```python
from build123d import *

# Parameters (mm, degrees)
SKETCH1_W                                    = 225
SKETCH1_H                                    = 47
SKETCH1_H_2                                  = 7
BOSS_EXTRUDE1_DEPTH                          = 3
SKETCH3_R                                    = 1.767766953
CUT_EXTRUDE1_DEPTH                           = 117.59974271
CHAMFER2_SIZE                                = 2
SKETCH2_W                                    = 225
SKETCH2_H                                    = 33
SKETCH2_R                                    = 15
CUT_EXTRUDE2_DEPTH                           = 0.2
FILLET1_R                                    = 3.5
CSK_FOR_M3_COUNTERSUNK_FLAT_HEAD_SCR_2_COUNT = 2
CSK_FOR_M3_COUNTERSUNK_FLAT_HEAD_SCR_2_PITCH = 47
CSK_FOR_M3_COUNTERSUNK_FLAT_HEAD_SCR_3_COUNT = 2
CSK_FOR_M3_COUNTERSUNK_FLAT_HEAD_SCR_3_PITCH = 223.00896843
CSK_FOR_M3_COUNTERSUNK_FLAT_HEAD_SCR_4_COUNT = 2
CSK_FOR_M3_COUNTERSUNK_FLAT_HEAD_SCR_4_PITCH = 218


with BuildPart() as part:
    # Sketch1 → Boss-Extrude1 (new body)
    with BuildSketch(Plane(origin=(0, 0, 0), x_dir=(1, 0, 0), z_dir=(0, 1, 0))):
        Rectangle(SKETCH1_W, SKETCH1_H)
        with Locations((0, -27)):
            Rectangle(SKETCH1_W, SKETCH1_H_2)
    extrude(amount=BOSS_EXTRUDE1_DEPTH)

    # Sketch3 → Cut-Extrude1 (cut, through all)
    with BuildSketch(Plane(origin=(0, 3, 0), x_dir=(1, 0, 0), z_dir=(0, 1, 0))):
        with Locations(Location((0, 15.5, 0), (0, 0, 270))):
            Circle(SKETCH3_R)
        with Locations(Location((45, 15.5, 0), (0, 0, 270))):
            Circle(SKETCH3_R)
        with Locations(Location((90, 15.5, 0), (0, 0, 270))):
            Circle(SKETCH3_R)
        with Locations(Location((-45, 15.5, 0), (0, 0, 270))):
            Circle(SKETCH3_R)
        with Locations(Location((-90, 15.5, 0), (0, 0, 270))):
            Circle(SKETCH3_R)
    extrude(amount=-CUT_EXTRUDE1_DEPTH, mode=Mode.SUBTRACT)

    # Chamfer2
    chamfer2_edges = [part.edges().sort_by_distance(p)[0] for p in [
        (-90, 3, -17.267766953),
        (-45, 3, -17.267766953),
        (90, 3, -17.267766953),
        (45, 3, -17.267766953),
        (0, 3, -17.267766953),
    ]]
    chamfer(chamfer2_edges, length=CHAMFER2_SIZE)

    # Sketch2 → Cut-Extrude2 (cut)
    # profile 1 of 6: a face of its own
    with BuildSketch(Plane(origin=(0, 3, 0), x_dir=(1, 0, 0), z_dir=(0, 1, 0))):
        with Locations((0, -7)):
            Rectangle(SKETCH2_W, SKETCH2_H)
        with Locations((-90, -7)):
            Circle(SKETCH2_R, mode=Mode.SUBTRACT)
        with Locations((-45, -7)):
            Circle(SKETCH2_R, mode=Mode.SUBTRACT)
        with Locations((0, -7)):
            Circle(SKETCH2_R, mode=Mode.SUBTRACT)
        with Locations((45, -7)):
            Circle(SKETCH2_R, mode=Mode.SUBTRACT)
        with Locations((90, -7)):
            Circle(SKETCH2_R, mode=Mode.SUBTRACT)
    # profile 2 of 6: a face of its own
    with BuildSketch(Plane(origin=(0, 3, 0), x_dir=(1, 0, 0), z_dir=(0, 1, 0))):
        with Locations((-90, -7)):
            Circle(SKETCH2_R)
    # profile 3 of 6: a face of its own
    with BuildSketch(Plane(origin=(0, 3, 0), x_dir=(1, 0, 0), z_dir=(0, 1, 0))):
        with Locations((-45, -7)):
            Circle(SKETCH2_R)
    # profile 4 of 6: a face of its own
    with BuildSketch(Plane(origin=(0, 3, 0), x_dir=(1, 0, 0), z_dir=(0, 1, 0))):
        with Locations((0, -7)):
            Circle(SKETCH2_R)
    # profile 5 of 6: a face of its own
    with BuildSketch(Plane(origin=(0, 3, 0), x_dir=(1, 0, 0), z_dir=(0, 1, 0))):
        with Locations((45, -7)):
            Circle(SKETCH2_R)
    # profile 6 of 6: a face of its own
    with BuildSketch(Plane(origin=(0, 3, 0), x_dir=(1, 0, 0), z_dir=(0, 1, 0))):
        with Locations((90, -7)):
            Circle(SKETCH2_R)
    extrude(amount=-CUT_EXTRUDE2_DEPTH, mode=Mode.SUBTRACT)

    # Fillet1
    fillet1_edges = [part.edges().sort_by_distance(p)[0] for p in [
        (112.5, 1.5, 30.5),
        (-112.5, 1.5, 30.5),
        (-112.5, 1.5, -23.5),
        (112.5, 1.5, -23.5),
    ]]
    fillet(fillet1_edges, radius=FILLET1_R)

    # Sketch5 → CSK for M3 Countersunk Flat Head Screw1 (revolve, cut)
    with BuildSketch(Plane(origin=(109, 3, -20), x_dir=(0, 0, 1), z_dir=(1, 0, 0))):
        Polygon((0, 0), (0, 3), (1.7, 3), (1.7, 1.55), (3.25, 0), align=None)
    csk_for_m3_countersunk_flat_head_screw1 = revolve(axis=Axis((109, 9.35, -20), (0, -1, 0)), mode=Mode.SUBTRACT)

    # CSK for M3 Countersunk Flat Head Scr 2: CSK for M3 Countersunk Flat Head Screw1 ×2
    with Locations(*[(0, 0, i * CSK_FOR_M3_COUNTERSUNK_FLAT_HEAD_SCR_2_PITCH) for i in range(1, CSK_FOR_M3_COUNTERSUNK_FLAT_HEAD_SCR_2_COUNT)]):
        add(csk_for_m3_countersunk_flat_head_screw1, mode=Mode.SUBTRACT)

    # CSK for M3 Countersunk Flat Head Scr 3: CSK for M3 Countersunk Flat Head Screw1 ×2
    with Locations(*[Vector(-0.977539161474997, 0, 0.21075385591433424) * (i * CSK_FOR_M3_COUNTERSUNK_FLAT_HEAD_SCR_3_PITCH) for i in range(1, CSK_FOR_M3_COUNTERSUNK_FLAT_HEAD_SCR_3_COUNT)]):
        add(csk_for_m3_countersunk_flat_head_screw1, mode=Mode.SUBTRACT)

    # CSK for M3 Countersunk Flat Head Scr 4: CSK for M3 Countersunk Flat Head Screw1 ×2
    with Locations(*[(-i * CSK_FOR_M3_COUNTERSUNK_FLAT_HEAD_SCR_4_PITCH, 0, 0) for i in range(1, CSK_FOR_M3_COUNTERSUNK_FLAT_HEAD_SCR_4_COUNT)]):
        add(csk_for_m3_countersunk_flat_head_screw1, mode=Mode.SUBTRACT)


solid = part.part
```
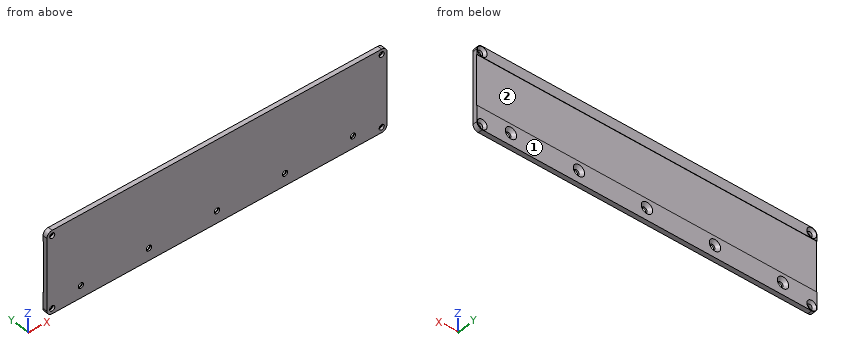
The model under review builds one solid part; all positions refer to its coordinate system, in mm. Face numbers are marked on the shaded views. Give positions to 0.01 mm unless a question says otherwise; leave off trailing zeros. Write each loop counter-clockwise with the first axis right and the second up, starting at its lowest first coordinate (ties: lowest second). Pieces come first, ordered by that corner, then holes. Notation, with made-up numbers: M 88,32 L 132,32 A25 cw 132,62 Z; hole C 3.25,3.5 d3. An arc over 180 degrees is marked long. Answer in a Markdown table with one row per item.
Item 1: Draft analysis for pull direction Z (two halves, no side actions). For the marked faces 1 and 2, state which applies: +Z half, -Z half, draft (parallel to the pull), parting line (faces both ways), or undercut.
Check sheet entries:
| item | result |
|---|---|
| face 1 | draft |
| face 2 | undercut |
Item 2: Add section B-B on y = 2.2. State how many separate pieces and enclosed holes the cut face has, plus the area to 3 significant figures.
Check sheet entries:
| item | result |
|---|---|
| separate pieces | 1 |
| enclosed holes | 9 |
| area | 11,900 mm2 |
Item 3: For line 1 along X through (y, z) = (0.55, -15.5); line 2 along Z through (x, y) = (-109, 0.6); line 3 along X through (y, z) = (2.05, -19.5) (3 decimals), list the stretches that pass through material, from the lowest coordinate up.
Check sheet entries:
| item | result |
|---|---|
| line 1 | -112.5 to -91.77, -88.23 to -46.77, -43.23 to -1.77, 1.77 to 43.23, 46.77 to 88.23, 91.77 to 112.5 |
| line 2 | -23.5 to -21.7, -18.3 to 25.3, 28.7 to 30.5 |
| line 3 | -112.5 to -111.245, -106.755 to 106.755, 111.245 to 112.5 |
Item 4: For P1, Ø1, axis at x = -81.5, z = 20, coming from the +Y side; P2, Ø3, axis at x = -109, z = -20, coming from the -Y side; P3, Ø4.5, axis at x = -90, z = -15.5, coming from the +Y side, all flat-tipped, find the tip position at first contact; note any pin that passes through.
Check sheet entries:
| item | result |
|---|---|
| P1 | y = 2.8 |
| P2 | through |
| P3 | y = 1.48 |
Item 5: Add section A-A on x = -22. Give the boundary of the cut face in (y, z), plus the area to 3 significant figures.
Check sheet entries:
| item | result |
|---|---|
| outline | M 0,-23.5 L 3,-23.5 L 3,-9.5 L 2.8,-9.5 L 2.8,23.5 L 3,23.5 L 3,30.5 L 0,30.5 Z |
| area | 155 mm2 |
